Geometry: final body of the model. Coordinates: model frame, mm. Give positions to 0.01 mm unless a question says otherwise; leave off trailing zeros. Write each loop counter-clockwise with the first axis right and the second up, starting at its lowest first coordinate (ties: lowest second). Pieces come first, ordered by that corner, then holes. Notation, with made-up numbers: (-24.75, -10) -> (29.25, -10) arc R7 cw to (29.25, 3) -> close; hole circle Ø3 at (65, 52). An arc over 180 degrees is marked (long way). Answer in a Markdown table with one row per item. Add a question column.
Item 1: Section query A-A on z = 5.5. Output: boundary loops of the cut face in (x, y).
Item 2: Section query C-C on x = -45.75. Output: boundary loops of the cut face in (y, z).
Item 3: Section query B-B on x = -54.5. Output: boundary loops of the cut face in (y, z), plus the area to 3 significant figures.
Item 4: Material intervals for probe 1 along Y at (x, z) = (-50.75, 0.5); probe 2 along Y at (x, z) = (-51.25, 5.25); probe 3 along X at (y, z) = (-37, 7), sorted ascending. Write a range as from..to.
Item 5: Draft query along X for faces 1 (the flat face through (-44.497, 0, 4)), 2 (the cylindrical face through (-50.365, 41.443, 4.19)), 3 (the flat face through (-56.497, 1, 4)), 4 (the cylindrical face through (-52.495, 0.532, 4.31)). Return one class per face: +X half, -X half, draft (parallel to the pull), parting line (faces both ways), or undercut.
Item 6: First-contact query: P1, Ø3.5, axis at x = -50.5, y = 0.44, coming from the +Z side; P2, Ø2, axis at x = -47.5, z = 6, coming from the -Y side. Flat tips, straight axial feed; report the tip coordinate or a pass-through.
```python
from build123d import *

# Parameters (mm, degrees)
F1_DEPTH = 8.5
F2_R     = 2
F3_DEPTH = 25


with BuildPart() as f1:
    # F0 (on Top) → F1 (new body)
    with BuildSketch(Plane.XY):
        with BuildLine():
            ThreePointArc((-44.496713, 35.444079), (-50.496713, 41.444079), (-56.496713, 35.444079))
            Line((-56.496713, 35.444079), (-56.496713, -34.555921))
            ThreePointArc((-56.496713, -34.555921), (-50.496713, -40.555921), (-44.496713, -34.555921))
            Line((-44.496713, -34.555921), (-44.496713, 35.444079))
        make_face()
    extrude(amount=F1_DEPTH)

    # F2 (on face) → F3 (cut)
    with BuildSketch(Plane.XY.offset(8.5)):
        with Locations((-50.496713, 0.444079)):
            Circle(F2_R)
    extrude(amount=-F3_DEPTH, mode=Mode.SUBTRACT)


solid = f1.part
```
Findings below:
| question | item | result |
|---|---|---|
| 1 | outline | (-56.5, -34.56) arc R6 ccw to (-44.5, -34.56) -> (-44.5, 35.44) arc R6 ccw to (-56.5, 35.44) -> close; hole circle Ø4 at (-50.5, 0.44) |
| 2 | outline | (-38.23, 0) -> (39.11, 0) -> (39.11, 8.5) -> (-38.23, 8.5) -> close |
| 3 | outline | (-39.03, 0) -> (39.91, 0) -> (39.91, 8.5) -> (-39.03, 8.5) -> close |
| 3 | area | 671 mm^2 |
| 4 | probe 1 | y = -40.55..-1.54, 2.43..41.44 |
| 4 | probe 2 | y = -40.51..-1.41, 2.3..41.4 |
| 4 | probe 3 | x = -55.98..-45.02 |
| 5 | face 1 | +X half |
| 5 | face 2 | parting line |
| 5 | face 3 | -X half |
| 5 | face 4 | undercut |
| 6 | P1 | passes through |
| 6 | P2 | stops at y = -40.21 |
